from build123d import *

# Parameters (mm, degrees)
BOSS_EXTRUDE1_DEPTH     = 41.275
CUT_EXTRUDE1_DEPTH      = 68.873747686
CUT_EXTRUDE1_DEPTH_BACK = 68.873747686
SKETCH2_R               = 25.4
CUT_EXTRUDE2_DEPTH      = 68.873747686
CUT_EXTRUDE2_DEPTH_BACK = 68.873747686
SKETCH3_R               = 3.2639
CUT_EXTRUDE3_DEPTH      = 68.87374786
CUT_EXTRUDE3_DEPTH_BACK = 68.87374786
SKETCH4_R               = 3.2639


with BuildPart() as part:
    # Sketch1 → Boss-Extrude1 (new body)
    with BuildSketch(Plane(origin=(0, 0, 0), x_dir=(-1, 0, 0), z_dir=(0, 1, 0))):
        with BuildLine():
            Line((-38.1, 0), (-38.1, -38.1))
            Line((-38.1, -38.1), (38.1, -38.1))
            Line((38.1, -38.1), (38.1, 0))
            ThreePointArc((38.1, 0), (0, 38.1), (-38.1, 0))
        make_face()
    extrude(amount=BOSS_EXTRUDE1_DEPTH)

    # Sketch2 → Cut-Extrude1 (cut, two sides: drawn at the far end of the back side and taken through both)
    with BuildSketch(Plane(origin=(0, 41.275, 0), x_dir=(-1, 0, 0), z_dir=(0, 1, 0)).offset(-CUT_EXTRUDE1_DEPTH_BACK)):
        with Locations(Location((0, 0, 0), (0, 0, 90))):
            Circle(SKETCH2_R)
    extrude(amount=CUT_EXTRUDE1_DEPTH + CUT_EXTRUDE1_DEPTH_BACK, mode=Mode.SUBTRACT)

    # Sketch3 → Cut-Extrude2 (cut, two sides: drawn at the far end of the back side and taken through both)
    with BuildSketch(Plane(origin=(0, 0, 0), x_dir=(0, 1, 0), z_dir=(0, 0, 1)).offset(-CUT_EXTRUDE2_DEPTH_BACK)):
        with Locations(Location((13.758333333, 0, 0), (0, 0, 270))):
            Circle(SKETCH3_R)
    extrude(amount=CUT_EXTRUDE2_DEPTH + CUT_EXTRUDE2_DEPTH_BACK, mode=Mode.SUBTRACT)

    # Sketch4 → Cut-Extrude3 (cut, two sides: drawn at the far end of the back side and taken through both)
    with BuildSketch(Plane.YZ.offset(-CUT_EXTRUDE3_DEPTH_BACK)):
        with Locations(Location((27.516666667, 0, 0), (0, 0, 270))):
            Circle(SKETCH4_R)
    extrude(amount=CUT_EXTRUDE3_DEPTH + CUT_EXTRUDE3_DEPTH_BACK, mode=Mode.SUBTRACT)


solid = part.part
Geometry check sheet. Reference: the model listing, model coordinates, mm. Round coordinates to 2 decimals unless told otherwise and drop trailing zeros. Order: outer loops, then holes, each group sorted by start corner. A loop starts at its lowest first (then second) coordinate and runs counter-clockwise, first axis right, second up. Notation, with made-up numbers: M -26.75,28 L 24.25,28 A22 cw 24.25,45 Z; hole C 9.25,-39 d10. An arc over 180 degrees is marked long. Answer in a Markdown table with one row per item. Add a question column.
Item 1: Sectioned sample at B-B, the plane z = 16.5. Enter the section's corners in (x, y) (3 decimals), plus the area to 3 significant figures.
Item 2: Sectioned sample at A-A, the plane x = 0. Enter the section's corners in (y, z) (3 decimals), plus the area to 3 significant figures.
Item 3: Draft check along Y on faces 1 (the face through (38.1, 20, -19)), 2 (the face through (-31.73, 24.33, 0.71)), 3 (the face through (-8, 0, -25)). Enter one of: released by +Y, released by -Y, zero draft, split by the parting line, or undercut.
Item 4: Sectioned sample at C-C, the plane y = 20. Enter the section's corners in (x, z), plus the area to 3 significant figures.
Item 5: Material ranges on L1, parallel to Y at x = 33, z = 0 (3 decimals); L2, parallel to X at y = 9, z = 0; L3, parallel to Z at x = -12.5, y = 40, recorded low to high. Write a range as [from, to].
Item 6: Sectioned sample at D-D, the plane x = -11. Enter the section's corners in (y, z) (3 decimals), plus the area to 3 significant figures.
Item 7: Depth check by flat-ended pin: pin 1 Ø12 at (y, z) = (37, 8.5) entering from +X; pin 2 Ø10.5 at (y, z) = (27.52, 0) entering from +X; pin 3 Ø3 at (x, y) = (6.5, 31) entering from +Z; pin 4 Ø5 at (y, z) = (37, 17) entering from +X. Enter the tip coordinate at first touch or a pass-through.
Filled in:
| question | item | result |
|---|---|---|
| 1 | outline | M -34.342,0 L -19.311,0 L -19.311,41.275 L -34.342,41.275 Z; M 19.311,0 L 34.342,0 L 34.342,41.275 L 19.311,41.275 Z |
| 1 | area | 1,240 mm² |
| 2 | outline | M 0,-38.1 L 10.494,-38.1 L 10.494,-25.4 L 0,-25.4 Z; M 0,25.4 L 10.494,25.4 L 10.494,38.1 L 0,38.1 Z; M 17.022,-38.1 L 41.275,-38.1 L 41.275,-25.4 L 17.022,-25.4 Z; M 17.022,25.4 L 41.275,25.4 L 41.275,38.1 L 17.022,38.1 Z |
| 2 | area | 883 mm² |
| 3 | face 1 | zero draft |
| 3 | face 2 | undercut |
| 3 | face 3 | released by -Y |
| 4 | outline | M -38.1,-38.1 L 38.1,-38.1 L 38.1,0 A38.1 ccw -38.1,0 Z; hole C 0,0 d50.8 |
| 4 | area | 3,160 mm² |
| 5 | L1 | y = [0, 24.253], [30.781, 41.275] |
| 5 | L2 | x = [-38.1, -25.4], [25.4, 38.1] |
| 5 | L3 | z = [-38.1, -22.11], [22.11, 35.99] |
| 6 | outline | M 0,-38.1 L 41.275,-38.1 L 41.275,-22.895 L 0,-22.895 Z; M 0,22.895 L 41.275,22.895 L 41.275,36.478 L 0,36.478 Z |
| 6 | area | 1,190 mm² |
| 7 | pin 1 | stops at x = 38.02 |
| 7 | pin 2 | stops at x = 38.1 |
| 7 | pin 3 | stops at z = 37.77 |
| 7 | pin 4 | stops at x = 35.23 |
